For this review, take the finished solid that the model builds, in its own axes (mm). A direction names the side the tool comes from. Coordinates: 2 decimals unless noted, no trailing zeros. Loops run counter-clockwise (first coordinate to the right, second up) from the corner with the lowest first, then second, coordinate; pieces in that order, holes last. Notation, with made-up numbers: (12.25, -21.5) -> (22.25, -21.5) arc R33 cw to (22.25, 13.5) -> close; hole circle Ø11 at (1.5, 17.25). An arc over 180 degrees is marked (long way). One line per item, written item: value.
from build123d import *

# Parameters (mm, degrees)
SKETCH_1_R      = 3.95
EXTRUDE_1_DEPTH = 6
SKETCH_3_R      = 4.5
SKETCH_2_R      = 3.95


with BuildPart() as part:
    # 스케치1 → 보스-돌출1 (new body)
    with BuildSketch(Plane.XY):
        Circle(SKETCH_1_R)
    extrude(amount=EXTRUDE_1_DEPTH)

    # 스케치3 → 로프트1 section 0
    with BuildSketch(Plane.XY.offset(8)):
        Circle(SKETCH_3_R)
    # 스케치2 → 로프트1 section 1
    with BuildSketch(Plane.XY.offset(6)):
        Circle(SKETCH_2_R)
    loft()

    # 스케치5 → 로프트2 section 0
    with BuildSketch(Plane.XY.offset(12)):
        with BuildLine():
            Line((0, -0.658032332), (0.569872716, -0.329016166))
            Line((0.569872716, -0.329016166), (0.569872716, 0.329016166))
            Line((0.569872716, 0.329016166), (0, 0.658032332))
            Line((0, 0.658032332), (-0.569872716, 0.329016166))
            Line((-0.569872716, 0.329016166), (-0.569872716, -0.329016166))
            Line((-0.569872716, -0.329016166), (0, -0.658032332))
        make_face()
    # 스케치4 for 로프트2 → 로프트2 section 1
    with BuildSketch(Plane.XY.offset(8)):
        with BuildLine():
            # circular arc as an exact rational Bezier (weights 1, cos(half-angle), 1)
            Bezier((0, -4.5), (2.598076211, -4.5), (3.897114317, -2.25), weights=[1, 0.866025404, 1])
            Bezier((3.897114317, -2.25), (5.196152423, 0), (3.897114317, 2.25), weights=[1, 0.866025404, 1])
            Bezier((3.897114317, 2.25), (2.598076211, 4.5), (0, 4.5), weights=[1, 0.866025404, 1])
            Bezier((0, 4.5), (-2.598076211, 4.5), (-3.897114317, 2.25), weights=[1, 0.866025404, 1])
            Bezier((-3.897114317, 2.25), (-5.196152423, 0), (-3.897114317, -2.25), weights=[1, 0.866025404, 1])
            Bezier((-3.897114317, -2.25), (-2.598076211, -4.5), (0, -4.5), weights=[1, 0.866025404, 1])
        make_face()
    loft()


solid = part.part
1. For faces 1 (the flat face through (0, 0, 0)), 2 (the cylindrical face through (-3.135, -2.404, 2.958)), list the 3-axis set-ups (+Z, -Z, +X, -X, +Y, -Y) from which the entire face can be reached by the end or side of a thin tool; tool diameter is ignored.
Return value:
face 1: -Z, +X, -X, +Y, -Y
face 2: -Z
2. Take a section at A-A, the plane z = 5.75. Give the boundary of the cut face in (x, y).
Return value:
outline: circle Ø7.9 at (0, 0)
3. To check wall thickness, follow probe 1 along Y at (x, z) = (-1, 1.5); probe 2 along Y at (x, z) = (2.75, 3.25); probe 3 along Z at (x, y) = (-1.25, 3). State the ranges of each line that lie inside material, in increasing order. Write a range as from..to.
Return value:
probe 1: y = -3.82..3.82
probe 2: y = -2.84..2.84
probe 3: z = 0..9.27
4. Insertion check: pin 1 Ø2 at (x, z) = (-0.5, 10) entering from +Y; pin 2 Ø1.5 at (y, z) = (-0.5, 5) entering from +X. Each pin has a flat end and moves straight along its axis. Give the tip position at first contact, or say it passes through.
Return value:
pin 1: stops at y = 3.5
pin 2: stops at x = 3.95
